The drawing under review shows one solid part. Ordinate dimensions are in mm from its lowest x, y, z. A direction names the side the tool comes from. Give positions to 0.01 mm unless a question says otherwise; leave off trailing zeros. Write each loop counter-clockwise with the first axis right and the second up, starting at its lowest first coordinate (ties: lowest second). Pieces come first, ordered by that corner, then holes. Notation, with made-up numbers: M -18,24 L 40,24 A15 cw 40,50 Z; hole C -25.75,81 d3. An arc over 180 degrees is marked long. Answer as a JSON object with one key per item and string values. Group by question number.
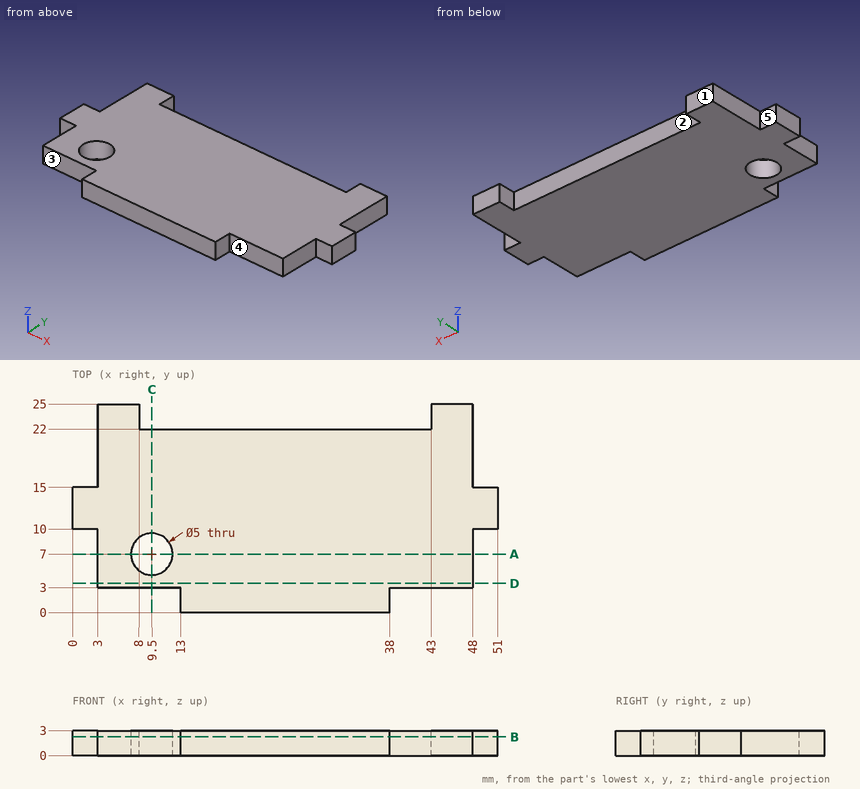
Item 1: To check wall thickness, follow probe 1 along Y at (x, z) = (9.5, 1.9); probe 2 along Y at (x, z) = (30, 2.2); probe 3 along X at (y, z) = (21, 2.5). State the ranges of each line that lie inside material, in increasing order.
Item 2: Consider section D-D (y = 3.5). Give the boundary of the cut face in (x, z).
Item 3: Draft analysis for pull direction X (two halves, no side actions). For the marked faces 1 and 2, state which applies: released by +X, released by -X, zero draft, split by the parting line, or undercut.
Item 4: Consider section C-C (x = 9.5). Give the boundary of the cut face in (y, z).
Item 5: Consider section B-B (z = 2.25). Give the boundary of the cut face in (x, y).
Item 6: Machinability: for the marked faces 3, 4 and 5, which of the approach directions +Z, -Z, +X, -X, +Y, -Y give a long, thin tool a straight path to every point of the face, cutting with its end or side? Answer none if there is none.
Item 7: Consider section A-A (y = 7). Give the boundary of the cut face in (x, z).
Item 8: Insertion check: P1, Ø1.5, axis at x = 49.5, z = 1, coming from the -Y side; P2, Ø1.5, axis at x = 9, y = 6.5, coming from the +Z side; P3, Ø0.9, axis at y = 18, z = 2, coming from the -X side; P4, Ø0.9, axis at x = 1.5, z = 1, coming from the +Y side. Each pin has a flat end and moves straight along its axis. Give the tip position at first contact, or say it passes through.
Result set:
{
 "1": {"probe 1": "y = 3 to 4.5, 9.5 to 22", "probe 2": "y = 0 to 22", "probe 3": "x = 3 to 48"},
 "2": {"outline": "M 3,0 L 48,0 L 48,3 L 3,3 Z"},
 "3": {"face 1": "zero draft", "face 2": "undercut"},
 "4": {"outline": "M 3,0 L 4.5,0 L 4.5,3 L 3,3 Z; M 9.5,0 L 22,0 L 22,3 L 9.5,3 Z"},
 "5": {"outline": "M 0,10 L 3,10 L 3,3 L 13,3 L 13,0 L 38,0 L 38,3 L 48,3 L 48,10 L 51,10 L 51,15 L 48,15 L 48,25 L 43,25 L 43,22 L 8,22 L 8,25 L 3,25 L 3,15 L 0,15 Z; hole C 9.5,7 d5"},
 "6": {"face 3": "+Z, -Z, -X, -Y", "face 4": "+Z, -Z, +X, -Y", "face 5": "+Z, -Z, -X, +Y"},
 "7": {"outline": "M 3,0 L 7,0 L 7,3 L 3,3 Z; M 12,0 L 48,0 L 48,3 L 12,3 Z"},
 "8": {"P1": "stops at y = 10", "P2": "passes through", "P3": "stops at x = 3", "P4": "stops at y = 15"}
}
